Verification items for the finished model (mm, model axes). A direction names the side the tool comes from. Give positions to 0.01 mm unless a question says otherwise; leave off trailing zeros. Loops run counter-clockwise (first coordinate to the right, second up) from the corner with the lowest first, then second, coordinate; pieces in that order, holes last. Notation, with made-up numbers: (23.25, 50.25) -> (39.25, 50.25) arc R13 ccw to (39.25, 71.25) -> close; hole circle Ø7 at (-14, -3.5). An arc over 180 degrees is marked (long way). Answer in a Markdown table with one row per item. Add a question column.
Q1. Section check A-A on z = 14.25. Enter the section's corners in (x, y).
Q2. Release check for a two-part mould opening along X. For faces 3 (the face through (2, -3, 30)), 4 (the face through (-7.7, -8.65, 14.79)), 5 (the face through (-30.276, 1.479, 14.79)) record: pulls with the +X half, pulls with the -X half, needs draft (parallel to the pull), parting line crosses it, or undercut.
Q3. Section check B-B on x = -3.5. Enter the section's corners in (y, z), and give its area (3 significant figures).
Q4. Gauge pin test, flat ends, axial feed: P1, Ø13.5, axis at y = 5.5, z = 17.5, coming from the -X side; P2, Ø1, axis at y = 12.5, z = 17, coming from the +X side; P3, Ø10, axis at y = -3.5, z = 9, coming from the -X side; P4, Ø12, axis at x = -22.5, y = 8, coming from the -Z side. Record the tip position at first contact, or that the pin passes through.
Q5. Set-up check for faces 1 (the face through (2, -16.266, 15)), 2 (the face through (-23, 17.234, 15)): record each of +Z, -Z, +X, -X, +Y, -Y from which the full face is reachable in a straight line by a thin tool's end or side.
Q6. Section check D-D on x = 28. Enter the section's corners in (y, z).
Q7. Section check C-C on y = 12. Enter the section's corners in (x, z).
Q8. Material ranges on probe 1 along X at (y, z) = (-4, 3); probe 2 along X at (y, z) = (-4.5, 18.75); probe 3 along Y at (x, z) = (4.5, 5.5), recorded low to high.
```python
from build123d import *

# Parameters (mm, degrees)
F2_DEPTH = 30
F4_DEPTH = 30
F6_DEPTH = 30


with BuildPart() as f2:
    # F1 (on face) → F2 (new body)
    with BuildSketch(Plane.XY):
        Polygon((-27.811348, 18.733989), (-32.811348, -16.266011), (37.188652, -16.266011), (37.188652, -16.031536), (32.188652, 18.733989), align=None)
    extrude(amount=F2_DEPTH)

    # F3 (on face) → F4 (join)
    with BuildSketch(Plane.XY):
        with BuildLine():
            Line((-32.811348, -16.266011), (37.188652, -16.266011))
            ThreePointArc((37.188652, -16.266011), (2.188652, -11.266011), (-32.811348, -16.266011))
        make_face()
    extrude(amount=F4_DEPTH)

    # F5 (on Top) → F6 (cut)
    with BuildSketch(Plane.XY):
        with BuildLine():
            ThreePointArc((-30.244943, -12.443307), (-25.051853, -11.198209), (-19.811348, -10.170808))
            Line((-19.811348, -10.170808), (-19.811348, 17.233989))
            Line((-19.811348, 17.233989), (-26.005329, 17.233989))
            Line((-26.005329, 17.233989), (-30.244943, -12.443307))
        make_face()
        with BuildLine():
            ThreePointArc((24.188652, -10.170808), (29.444778, -11.201613), (34.653178, -12.451413))
            Line((34.653178, -12.451413), (30.383804, 17.233989))
            Line((30.383804, 17.233989), (24.188652, 17.233989))
            Line((24.188652, 17.233989), (24.188652, -10.170808))
        make_face()
        with BuildLine():
            ThreePointArc((3.688652, -8.2748), (11.959086, -8.639451), (20.188652, -9.537955))
            Line((20.188652, -9.537955), (20.188652, 17.233989))
            Line((20.188652, 17.233989), (3.688652, 17.233989))
            Line((3.688652, 17.233989), (3.688652, -8.2748))
        make_face()
        with BuildLine():
            ThreePointArc((-15.811348, -9.537955), (-7.581783, -8.639451), (0.688652, -8.2748))
            Line((0.688652, -8.2748), (0.688652, 17.233989))
            Line((0.688652, 17.233989), (-15.811348, 17.233989))
            Line((-15.811348, 17.233989), (-15.811348, -9.537955))
        make_face()
    extrude(amount=F6_DEPTH, mode=Mode.SUBTRACT)


solid = f2.part
```
Taken from the geometry:
| question | item | result |
|---|---|---|
| 1 | outline | (-32.81, -16.27) -> (37.19, -16.27) -> (37.19, -16.03) -> (32.19, 18.73) -> (-27.81, 18.73) -> close; hole (-30.24, -12.44) arc R128 cw to (-19.81, -10.17) -> (-19.81, 17.23) -> (-26.01, 17.23) -> close; hole (-15.81, -9.54) arc R128 cw to (0.69, -8.27) -> (0.69, 17.23) -> (-15.81, 17.23) -> close; hole (3.69, -8.27) arc R128 cw to (20.19, -9.54) -> (20.19, 17.23) -> (3.69, 17.23) -> close; hole (24.19, -10.17) arc R128 cw to (34.65, -12.45) -> (30.38, 17.23) -> (24.19, 17.23) -> close |
| 2 | face 3 | needs draft |
| 2 | face 4 | undercut |
| 2 | face 5 | pulls with the -X half |
| 3 | outline | (-16.27, 0) -> (-8.39, 0) -> (-8.39, 30) -> (-16.27, 30) -> close; (17.23, 0) -> (18.73, 0) -> (18.73, 30) -> (17.23, 30) -> close |
| 3 | area | 281 mm² |
| 4 | P1 | stops at x = -30.67 |
| 4 | P2 | stops at x = 33.16 |
| 4 | P3 | stops at x = -31.7 |
| 4 | P4 | stops at z = 0 |
| 5 | face 1 | +Z, -Z, +X, -X, -Y |
| 5 | face 2 | +Z, -Z |
| 6 | outline | (-16.27, 0) -> (-10.9, 0) -> (-10.9, 30) -> (-16.27, 30) -> close; (17.23, 0) -> (18.73, 0) -> (18.73, 30) -> (17.23, 30) -> close |
| 7 | outline | (-28.77, 0) -> (-26.75, 0) -> (-26.75, 30) -> (-28.77, 30) -> close; (-19.81, 0) -> (-15.81, 0) -> (-15.81, 30) -> (-19.81, 30) -> close; (0.69, 0) -> (3.69, 0) -> (3.69, 30) -> (0.69, 30) -> close; (20.19, 0) -> (24.19, 0) -> (24.19, 30) -> (20.19, 30) -> close; (31.14, 0) -> (33.16, 0) -> (33.16, 30) -> (31.14, 30) -> close |
| 8 | probe 1 | x = -31.06 to -29.04, -19.81 to -15.81, 0.69 to 3.69, 20.19 to 24.19, 33.44 to 35.46 |
| 8 | probe 2 | x = -31.13 to -29.11, -19.81 to -15.81, 0.69 to 3.69, 20.19 to 24.19, 33.51 to 35.53 |
| 8 | probe 3 | y = -16.27 to -8.29, 17.23 to 18.73 |
